```python
from build123d import *

# Parameters (mm, degrees)
SKETCH1_W           = 430
SKETCH1_H           = 190
SKETCH1_R           = 6
BOSS_EXTRUDE1_DEPTH = 6
FILLET1_R           = 95


with BuildPart() as part:
    # Sketch1 → Boss-Extrude1 (new body)
    with BuildSketch(Plane.XY):
        Rectangle(SKETCH1_W, SKETCH1_H)
        with Locations((-145, 52.92)):
            Circle(SKETCH1_R, mode=Mode.SUBTRACT)
        with Locations((45, 52.92)):
            Circle(SKETCH1_R, mode=Mode.SUBTRACT)
        with Locations((45, -52.92)):
            Circle(SKETCH1_R, mode=Mode.SUBTRACT)
        with Locations((-145, -52.92)):
            Circle(SKETCH1_R, mode=Mode.SUBTRACT)
    extrude(amount=BOSS_EXTRUDE1_DEPTH)

    # Fillet1
    fillet1_edges = [part.edges().sort_by_distance(p)[0] for p in [
        (-215, -95, 3),
        (-215, 95, 3),
    ]]
    fillet(fillet1_edges, radius=FILLET1_R - 0.0001)  # a hair under: the kernel refuses the full size


solid = part.part
```
Here's how the part is built. I have some questions about the finished solid (model axes, mm). Coordinates: 2 decimals unless noted, no trailing zeros. Order: outer loops, then holes, each group sorted by start corner. A loop starts at its lowest first (then second) coordinate and runs counter-clockwise, first axis right, second up.
1) Will these pins go through, and if not, where does the flat tip stop? pin 1 (2 mm diameter, centred on y = 52.5, z = 2.5, fed in from -X); pin 2 (3 mm diameter, centred on y = -56, z = 5, fed in from -X).
2) Imagine slicing it at B-B on x = 45. List the corners of the cut face in (y, z) for me, and give its area (3 significant figures).
3) Imagine slicing it at C-C on y = 52.92. List the corners of the cut face in (x, z) for me.
4) We'd pull the mould along X, two halves only. Please class faces 1 (the face through (40.24, -56.57, 2.96)), 2 (the face through (-187.91, -66.43, 3.04)), 3 (the face through (-3, 1, 6)): +X half, -X half, draft (parallel to the pull), parting line (faces both ways), or undercut.
5) Imagine slicing it at D-D on y = -71.5. List the corners of the cut face in (x, z) for me.
6) Imagine slicing it at A-A on z = 1.15. State how many separate pieces and enclosed holes the cut face has, and give its area (3 significant figures).
7) I need wall thicknesses on line 1 (Y direction, x = 45, z = 4.65); line 2 (X direction, y = 1.5, z = 1.8); line 3 (X direction, y = -29.5, z = 1.8). Which ranges of each line are inside material? Lowest first, please.
Response values:
1. pin 1: stops at x = -199.83
1. pin 2: stops at x = -197.81
2. outline: (-95, 0) - (-58.92, 0) - (-58.92, 6) - (-95, 6) - close; (-46.92, 0) - (46.92, 0) - (46.92, 6) - (-46.92, 6) - close; (58.92, 0) - (95, 0) - (95, 6) - (58.92, 6) - close
2. area: 996 mm2
3. outline: (-198.9, 0) - (-151, 0) - (-151, 6) - (-198.9, 6) - close; (-139, 0) - (39, 0) - (39, 6) - (-139, 6) - close; (51, 0) - (215, 0) - (215, 6) - (51, 6) - close
4. face 1: undercut
4. face 2: -X half
4. face 3: draft
5. outline: (-182.55, 0) - (215, 0) - (215, 6) - (-182.55, 6) - close
6. separate pieces: 1
6. enclosed holes: 4
6. area: 77,400 mm2
7. line 1: y = -95 to -58.92, -46.92 to 46.92, 58.92 to 95
7. line 2: x = -214.99 to 215
7. line 3: x = -210.3 to 215
